Geometry check sheet. Reference: the model listing, model coordinates, mm. Give positions to 0.01 mm unless a question says otherwise; leave off trailing zeros. Write each loop counter-clockwise with the first axis right and the second up, starting at its lowest first coordinate (ties: lowest second). Pieces come first, ordered by that corner, then holes. Notation, with made-up numbers: M -10,-1 L 25,-1 A17 cw 25,8 Z; hole C -21,-28 d1. An arc over 180 degrees is marked long. Use one line per item in the form item = value. Start each with the question number.
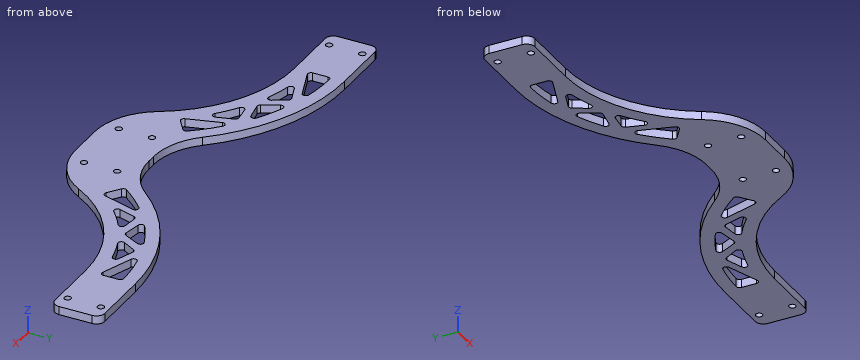
```python
from build123d import *

# Parameters (mm, degrees)
ESQUISSE1_R        = 2
BOSS_EXTRU_1_DEPTH = 5
CONG_1_R           = 5
CONG_2_R           = 40
CONG_3_R           = 2


with BuildPart() as part:
    # Esquisse1 → Boss.-Extru.1 (new body)
    with BuildSketch(Plane.XY):
        with BuildLine():
            Line((-37.5, 0), (37.5, 0))
            ThreePointArc((37.5, 0), (67.945941561, 45.786768838), (120, 63.5))
            Line((120, 63.5), (160, 63.5))
            Line((160, 63.5), (160, 93.5))
            Line((160, 93.5), (120, 93.5))
            ThreePointArc((120, 93.5), (64.453511348, 79.243999919), (22.637791694, 40))
            Line((22.637791694, 40), (-22.637791694, 40))
            ThreePointArc((-22.637791694, 40), (-64.453511348, 79.243999919), (-120, 93.5))
            Line((-120, 93.5), (-160, 93.5))
            Line((-160, 93.5), (-160, 63.5))
            Line((-160, 63.5), (-120, 63.5))
            ThreePointArc((-120, 63.5), (-67.945941561, 45.786768838), (-37.5, 0))
        make_face()
        with Locations((20, 30)):
            Circle(ESQUISSE1_R, mode=Mode.SUBTRACT)
        with Locations((-20, 30)):
            Circle(ESQUISSE1_R, mode=Mode.SUBTRACT)
        with Locations((-20, 10)):
            Circle(ESQUISSE1_R, mode=Mode.SUBTRACT)
        with Locations((20, 10)):
            Circle(ESQUISSE1_R, mode=Mode.SUBTRACT)
        with Locations((150, 88.5)):
            Circle(ESQUISSE1_R, mode=Mode.SUBTRACT)
        with Locations((150, 68.5)):
            Circle(ESQUISSE1_R, mode=Mode.SUBTRACT)
        with Locations((-150, 88.5)):
            Circle(ESQUISSE1_R, mode=Mode.SUBTRACT)
        with Locations((-150, 68.5)):
            Circle(ESQUISSE1_R, mode=Mode.SUBTRACT)
        with BuildLine():
            Line((120, 85.5), (120, 71.5))
            Line((120, 71.5), (91.912412909, 81.760105686))
            ThreePointArc((91.912412909, 81.760105686), (105.832260607, 84.560918666), (120, 85.5))
        make_face(mode=Mode.SUBTRACT)
        with BuildLine():
            Line((44.869226881, 33.548751393), (33.600720018, 41.856624351))
            ThreePointArc((33.600720018, 41.856624351), (42.763993121, 52.702874362), (53.278657874, 62.244810141))
            Line((53.278657874, 62.244810141), (44.869226881, 33.548751393))
        make_face(mode=Mode.SUBTRACT)
        with BuildLine():
            Line((52.630031511, 42.764858585), (58.158997811, 61.631716745))
            Line((58.158997811, 61.631716745), (74.382302486, 59.593661799))
            ThreePointArc((74.382302486, 59.593661799), (62.882968201, 51.984783256), (52.630031511, 42.764858585))
        make_face(mode=Mode.SUBTRACT)
        with BuildLine():
            Line((59.726445752, 66.980423245), (76.611394643, 64.052400369))
            Line((76.611394643, 64.052400369), (84.274506387, 79.380529263))
            ThreePointArc((84.274506387, 79.380529263), (71.601705042, 73.969909454), (59.726445752, 66.980423245))
        make_face(mode=Mode.SUBTRACT)
        with BuildLine():
            Line((81.522990402, 63.200679417), (89.509798834, 77.468130963))
            Line((89.509798834, 77.468130963), (107.976603852, 70.722397677))
            ThreePointArc((107.976603852, 70.722397677), (94.471255289, 67.941160205), (81.522990402, 63.200679417))
        make_face(mode=Mode.SUBTRACT)
        with BuildLine():
            Line((-120, 85.5), (-120, 71.5))
            Line((-120, 71.5), (-91.912412909, 81.760105686))
            ThreePointArc((-91.912412909, 81.760105686), (-105.832260607, 84.560918666), (-120, 85.5))
        make_face(mode=Mode.SUBTRACT)
        with BuildLine():
            Line((-89.509798834, 77.468130963), (-107.976603852, 70.722397677))
            ThreePointArc((-107.976603852, 70.722397677), (-94.471255289, 67.941160205), (-81.522990402, 63.200679417))
            Line((-81.522990402, 63.200679417), (-89.509798834, 77.468130963))
        make_face(mode=Mode.SUBTRACT)
        with BuildLine():
            Line((-76.611394643, 64.052400369), (-84.274506387, 79.380529263))
            ThreePointArc((-84.274506387, 79.380529263), (-71.601705042, 73.969909454), (-59.726445752, 66.980423245))
            Line((-59.726445752, 66.980423245), (-76.611394643, 64.052400369))
        make_face(mode=Mode.SUBTRACT)
        with BuildLine():
            Line((-58.158997811, 61.631716745), (-74.382302486, 59.593661799))
            ThreePointArc((-74.382302486, 59.593661799), (-62.882968201, 51.984783256), (-52.630031511, 42.764858585))
            Line((-52.630031511, 42.764858585), (-58.158997811, 61.631716745))
        make_face(mode=Mode.SUBTRACT)
        with BuildLine():
            Line((-44.869226881, 33.548751393), (-33.600720018, 41.856624351))
            ThreePointArc((-33.600720018, 41.856624351), (-42.763993121, 52.702874362), (-53.278657874, 62.244810141))
            Line((-53.278657874, 62.244810141), (-44.869226881, 33.548751393))
        make_face(mode=Mode.SUBTRACT)
    extrude(amount=BOSS_EXTRU_1_DEPTH)

    # Congé1
    cong_1_edges = [part.edges().sort_by_distance(p)[0] for p in [
        (160, 93.5, 2.5),
        (160, 63.5, 2.5),
        (-160, 63.5, 2.5),
        (-160, 93.5, 2.5),
    ]]
    fillet(cong_1_edges, radius=CONG_1_R)

    # Congé2
    cong_2_edges = [part.edges().sort_by_distance(p)[0] for p in [
        (-22.637791694, 40, 2.5),
        (22.637791694, 40, 2.5),
        (37.5, 0, 2.5),
        (-37.5, 0, 2.5),
    ]]
    fillet(cong_2_edges, radius=CONG_2_R)

    # Congé3
    cong_3_edges = [part.edges().sort_by_distance(p)[0] for p in [
        (-58.158997811, 61.631716745, 2.5),
        (-74.382302486, 59.593661799, 2.5),
        (-52.630031511, 42.764858585, 2.5),
        (-76.611394643, 64.052400369, 2.5),
        (-59.726445752, 66.980423245, 2.5),
        (-84.274506387, 79.380529263, 2.5),
        (-120, 71.5, 2.5),
        (-91.912412909, 81.760105686, 2.5),
        (-120, 85.5, 2.5),
        (89.509798834, 77.468130963, 2.5),
        (81.522990402, 63.200679417, 2.5),
        (107.976603852, 70.722397677, 2.5),
        (44.869226881, 33.548751393, 2.5),
        (53.278657874, 62.244810141, 2.5),
        (33.600720018, 41.856624351, 2.5),
        (59.726445752, 66.980423245, 2.5),
        (76.611394643, 64.052400369, 2.5),
        (84.274506387, 79.380529263, 2.5),
        (91.912412909, 81.760105686, 2.5),
        (120, 71.5, 2.5),
        (120, 85.5, 2.5),
        (74.382302486, 59.593661799, 2.5),
        (58.158997811, 61.631716745, 2.5),
        (52.630031511, 42.764858585, 2.5),
        (-81.522990402, 63.200679417, 2.5),
        (-89.509798834, 77.468130963, 2.5),
        (-107.976603852, 70.722397677, 2.5),
        (-53.278657874, 62.244810141, 2.5),
        (-44.869226881, 33.548751393, 2.5),
        (-33.600720018, 41.856624351, 2.5),
    ]]
    fillet(cong_3_edges, radius=CONG_3_R)


solid = part.part
```
(1) Thickness scan on probe 1 along Y at (x, z) = (20, 1.1); probe 2 along Y at (x, z) = (-150, 2.95); probe 3 along Y at (x, z) = (1.5, 4.35). Record the ranges inside material, lowest first. Write a range as [from, to].
(2) Sectioned sample at D-D, the plane x = -28. Record the boundary of the cut face in (y, z), plus the area to 3 significant figures.
(3) Depth check by flat-ended pin: pin 1 (1 mm diameter, centred on x = -103.5, z = 1.5, fed in from +Y); pin 2 (2 mm diameter, centred on x = -42, z = 2.5, fed in from -Y). Enter the tip coordinate at first touch or a pass-through.
(4) Sectioned sample at C-C, the plane y = 16. Record the boundary of the cut face in (x, z).
(5) Sectioned sample at A-A, the plane x = -109. Record the boundary of the cut face in (y, z).
(6) Sectioned sample at B-B, the plane z = 3.15. State how many separate pieces and enclosed holes the cut face has, plus the area to 3 significant figures.
Numbers:
q1.probe_1 = [1.03, 8], [12, 28], [32, 43.93]
q1.probe_2 = [63.5, 66.5], [70.5, 86.5], [90.5, 93.5]
q1.probe_3 = [0, 40]
q2.outline = M 3.8,0 L 49.02,0 L 49.02,5 L 3.8,5 Z
q2.area = 226 mm2
q3.pin_1 = 92.38
q3.pin_2 = 13.57
q4.outline = M -42.98,0 L 42.98,0 L 42.98,5 L -42.98,5 Z
q5.outline = M 62.79,0 L 75.52,0 L 75.52,5 L 62.79,5 Z; M 84.93,0 L 92.97,0 L 92.97,5 L 84.93,5 Z
q6.separate_pieces = 1
q6.enclosed_holes = 18
q6.area = 9,760 mm2
